Autodesk Inventor part; units mm, degrees
ref_plane "YZ Plane" through (0, 0, 0) normal (1, 0, 0) x (0, 1, 0)
ref_plane "XZ Plane" through (0, 0, 0) normal (0, 1, 0) x (-1, 0, 0)
ref_plane "XY Plane" through (0, 0, 0) normal (0, 0, 1) x (1, 0, 0)
sketch "Эскиз1" plane through (0, 0, 0) normal (0, 0, 1) x (1, 0, 0)
  line L0 (-13.4163, 13.7539) -> (26.5837, 13.7539)
  line L1 (26.5837, 13.7539) -> (26.5837, -16.2461)
  line L2 (26.5837, -16.2461) -> (-13.4163, -16.2461)
  line L3 (-13.4163, -16.2461) -> (-13.4163, 13.7539)
  point P0 (0, 0)
  dimension "d0" = 40
  dimension "d1" = 30
extrude "Выдавливание1" add sketch "Эскиз1" along normal blind 8.3
sketch "Эскиз2" plane through (-13.4163, -16.2461, 0) normal (-1, 0, 0) x (0, 0, 1)
  line L0 (3, 6.5) -> (3.5, 6.5)
  line L1 (3.5, 6.5) -> (3.5, 10.5)
  line L2 (3.5, 10.5) -> (3, 10.5)
  line L3 (3, 10.5) -> (3, 6.5)
  line L4 (3, 19.5) -> (3.5, 19.5)
  line L5 (3.5, 19.5) -> (3.5, 23.5)
  line L6 (3.5, 23.5) -> (3, 23.5)
  line L7 (3, 23.5) -> (3, 19.5)
  line L8 (0, 0) -> (8.3, 0)
  line L9 (0, 30) -> (0, 0)
  point P0 (0, 16.2461)
  dimension "d4" = 4
  dimension "d5" = 4
  dimension "d6" = 0.5
  dimension "d7" = 0.5
  dimension "d8" = 9
  dimension "d9" = 6.5
  dimension "d10" = 3
extrude "Выдавливание2" add sketch "Эскиз2" along normal blind 4
fillet "Сопряжение1" radius 2 12 edges at (6.5837, 13.7539, 8.3) (6.5837, 13.7539, 0) (6.5837, -16.2461, 8.3) (6.5837, -16.2461, 0) (26.5837, -1.2461, 0) (26.5837, -1.2461, 8.3) (26.5837, -16.2461, 4.15) (-13.4163, -1.2461, 0) (-13.4163, -16.2461, 4.15) (-13.4163, 13.7539, 4.15) (-13.4163, -1.2461, 8.3) (26.5837, 13.7539, 4.15)
properties part number "803048" material "Алюминий 6061"
Work out the finished part from the listing and answer in its coordinate system (mm). A direction names the side the tool comes from. Give positions to 0.01 mm unless a question says otherwise; leave off trailing zeros. Loops run counter-clockwise (first coordinate to the right, second up) from the corner with the lowest first, then second, coordinate; pieces in that order, holes last. Notation, with made-up numbers: (60, -9) - (111, -9) arc R22 cw to (111, 14) - close; hole circle Ø4 at (-28.5, -31.75). An arc over 180 degrees is marked (long way). Use CSV: the item, a comma, the result in double quotes. Start each with the question number.
(1) Determine the mould class of faces 4 (the face through (-12.846, -1.064, 7.699)), 5 (the face through (-15, 5, 3.5)), 6 (the face through (25.98, -15.68, 4.18)) for opening direction X: released by +X, released by -X, zero draft, split by the parting line, or undercut.
(2) Find section C-C, the plane y = -0.25. Determine the outline of the cut face in (x, z), plus the area to 3 significant figures.
(3) A tool of negligible diameter and unlimited length cuts with its end or side. For faces 1 (the face through (-12.8, 13.2, 4.2)), 2 (the face through (-15, -8, 3.5)), 3 (the face through (-15, 5, 3)), from which of +Z, -Z, +X, -X, +Y, -Y can it reach the whole face along a straight path? Write none if from no direction.
(4) Find section A-A, the plane z = 5. Determine the outline of the cut face in (x, y), plus the area to 3 significant figures.
(5) Find section B-B, the plane y = -7.5. Determine the outline of the cut face in (x, z).
(6) Find the intervals of material crossed by L1, parallel to X at y = -9.5, z = 4.25; L2, parallel to Y at x = -0.5, z = 6.5; L3, parallel to X at y = -1, z = 1, in increasing order.
(7) Each of these flat-tipped pins is pushed along its axis until it touches: pin 1 (2 mm diameter, centred on x = -16, y = 5.5, fed in from +Z); pin 2 (4.5 mm diameter, centred on x = -15, y = -8, fed in from -Z); pin 3 (0.6 mm diameter, centred on x = -15, z = 3.5, fed in from -Y). Where does it stop, or does it pass through?
Results found:
1,face 4,"released by -X"
1,face 5,"zero draft"
1,face 6,"released by +X"
2,outline,"(-13.42, 2) arc R2 ccw to (-11.42, 0) - (24.58, 0) arc R2 ccw to (26.58, 2) - (26.58, 6.3) arc R2 ccw to (24.58, 8.3) - (-11.42, 8.3) arc R2 ccw to (-13.42, 6.3) - close"
2,area,"329 mm^2"
3,face 1,"+Z, -Z, -X, +Y"
3,face 2,"+Z, -X, +Y, -Y"
3,face 3,"-Z, -X, +Y, -Y"
4,outline,"(-13.42, -14.25) arc R2 ccw to (-11.42, -16.25) - (24.58, -16.25) arc R2 ccw to (26.58, -14.25) - (26.58, 11.75) arc R2 ccw to (24.58, 13.75) - (-11.42, 13.75) arc R2 ccw to (-13.42, 11.75) - close"
4,area,"1,200 mm^2"
5,outline,"(-17.42, 3) - (-13.42, 3) - (-13.42, 2) arc R2 ccw to (-11.42, 0) - (24.58, 0) arc R2 ccw to (26.58, 2) - (26.58, 6.3) arc R2 ccw to (24.58, 8.3) - (-11.42, 8.3) arc R2 ccw to (-13.42, 6.3) - (-13.42, 3.5) - (-17.42, 3.5) - close"
6,L1,"-13.42 to 26.58"
6,L2,"-16.24 to 13.74"
6,L3,"-13.15 to 26.32"
7,pin 1,"z = 3.5"
7,pin 2,"z = 0.51"
7,pin 3,"y = -9.75"
